The model under review builds one solid part; all positions refer to its coordinate system, in mm. A direction names the side the tool comes from. Coordinates: 2 decimals unless noted, no trailing zeros. Loops run counter-clockwise (first coordinate to the right, second up) from the corner with the lowest first, then second, coordinate; pieces in that order, holes last. Notation, with made-up numbers: M 58.25,-20.75 L 87.25,-20.75 A26 ccw 87.25,-3.75 Z; hole C -11,41 d8. An arc over 180 degrees is marked long. Use one line per item in the form item = value.
```python
from build123d import *

# Parameters (mm, degrees)
ESQUISSE1_R        = 105
ESQUISSE1_R_2      = 8
BOSS_EXTRU_1_DEPTH = 1
CONG_1_R           = 5


with BuildPart() as part:
    # Esquisse1 → Boss.-Extru.1 (new body)
    with BuildSketch(Plane.XY):
        Circle(ESQUISSE1_R)
        with BuildLine():
            Line((95.569858419, 16.595245155), (76.894171459, 11.591109915))
            ThreePointArc((76.894171459, 11.591109915), (68, 0), (76.894171459, -11.591109915))
            Line((76.894171459, -11.591109915), (95.569858419, -16.595245155))
            ThreePointArc((95.569858419, -16.595245155), (48.5, -84.004464167), (-33.413025324, -91.063547804))
            Line((-33.413025324, -91.063547804), (-28.408890085, -72.387860844))
            ThreePointArc((-28.408890085, -72.387860844), (-34, -58.889727457), (-48.485281374, -60.796750929))
            Line((-48.485281374, -60.796750929), (-62.156833095, -74.46830265))
            ThreePointArc((-62.156833095, -74.46830265), (-97, 0), (-62.156833096, 74.46830265))
            Line((-62.156833096, 74.46830265), (-48.485281374, 60.796750929))
            ThreePointArc((-48.485281374, 60.796750929), (-34, 58.889727457), (-28.408890085, 72.387860844))
            Line((-28.408890085, 72.387860844), (-33.413025324, 91.063547804))
            ThreePointArc((-33.413025324, 91.063547804), (48.5, 84.004464167), (95.569858419, 16.595245155))
        make_face(mode=Mode.SUBTRACT)
        with Locations((80, 0)):
            Circle(ESQUISSE1_R_2, mode=Mode.SUBTRACT)
        with Locations((-40, 69.282032303)):
            Circle(ESQUISSE1_R_2, mode=Mode.SUBTRACT)
        with Locations((-40, -69.282032303)):
            Circle(ESQUISSE1_R_2, mode=Mode.SUBTRACT)
    extrude(amount=BOSS_EXTRU_1_DEPTH)

    # Congé1
    cong_1_edges = [part.edges().sort_by_distance(p)[0] for p in [
        (-62.156833096, 74.46830265, 0.5),
        (-62.156833095, -74.46830265, 0.5),
        (-33.413025324, -91.063547804, 0.5),
        (95.569858419, -16.595245155, 0.5),
        (95.569858419, 16.595245155, 0.5),
        (-33.413025324, 91.063547804, 0.5),
    ]]
    fillet(cong_1_edges, radius=CONG_1_R)


solid = part.part
```
1. Add section D-D (z = 0.3). State the section outline as (x, y) points.
Response values:
outline = C 0,0 d210; hole M -65.77,-71.3 A5 ccw -58.85,-71.16 L -48.49,-60.8 A12 cw -28.41,-72.39 L -32.2,-86.54 A5 ccw -28.86,-92.61 A97 ccw 94.63,-21.31 A5 ccw 91.05,-15.38 L 76.89,-11.59 A12 cw 76.89,11.59 L 91.05,15.38 A5 ccw 94.63,21.31 A97 ccw -28.86,92.61 A5 ccw -32.2,86.54 L -28.41,72.39 A12 cw -48.49,60.8 L -58.85,71.16 A5 ccw -65.77,71.3 A97 ccw Z; hole C -40,-69.28 d16; hole C -40,69.28 d16; hole C 80,0 d16
2. Add section B-B (x = 0). State the section outline as (y, z) points.
Response values:
outline = M -105,0 L -97,0 L -97,1 L -105,1 Z; M 97,0 L 105,0 L 105,1 L 97,1 Z
3. Add section C-C (x = -40). State the section outline as (y, z) points.
Response values:
outline = M -97.08,0 L -77.28,0 L -77.28,1 L -97.08,1 Z; M -61.28,0 L -57.28,0 L -57.28,1 L -61.28,1 Z; M 57.28,0 L 61.28,0 L 61.28,1 L 57.28,1 Z; M 77.28,0 L 97.08,0 L 97.08,1 L 77.28,1 Z
4. The part is to be moulded in two halves that separate along X. For faces 3 (the face through (-34.191, 58.782, 0.493)), 4 (the face through (-32, -62, 0)), 5 (the face through (-33.81, -59, 0.49)), 6 (the face through (100.15, 31.54, 0.49)), say which applies: pulls with the +X half, pulls with the -X half, needs draft (parallel to the pull), parting line crosses it, or undercut.
Response values:
face_3 = undercut
face_4 = needs draft
face_5 = undercut
face_6 = parting line crosses it
5. Wall thickness on line 1 along X through (y, z) = (-61, 0.4); line 2 along Y through (x, z) = (-40, 0.6); line 3 along Y through (x, z) = (69, 0.8): over which ranges is each line inside the solid? List them lowest first. Write a range as from..to.
Response values:
line_1 = -85.46..-75.42, -48.69..-31.32, 75.42..85.46
line_2 = -97.08..-77.28, -61.28..-57.28, 57.28..61.28, 77.28..97.08
line_3 = -79.15..-68.18, -4.8..4.8, 68.18..79.15
6. Add section A-A (y = 0). State the section outline as (x, z) points, then the cut area to 3 significant figures.
Response values:
outline = M -105,0 L -97,0 L -97,1 L -105,1 Z; M 68,0 L 72,0 L 72,1 L 68,1 Z; M 88,0 L 105,0 L 105,1 L 88,1 Z
area = 29.0 mm^2
7. Insertion check: P1, Ø18.5, axis at x = 80, y = 0, coming from the +Z side. The pin has a flat end and moves straight along its axis. Give the tip position at first contact, or say it passes through.
Response values:
P1 = 1
8. Machinability: for faces 1 (the face through (-53.74, 66.05, 0.49)), 2 (the face through (-32, -62, 1)), which of the approach directions +Z, -Z, +X, -X, +Y, -Y give a long, thin tool a straight path to every point of the face, cutting with its end or side? Answer none if there is none.
Response values:
face_1 = +Z, -Z
face_2 = +Z, +X, -X, +Y, -Y
